from build123d import *

# Parameters (mm, degrees)
F0_W     = 18.8
F0_H     = 22.5
F1_DEPTH = 40


with BuildPart() as f1:
    # F0 (on Top) → F1 (new body)
    with BuildSketch(Plane.XY):
        Rectangle(F0_W, F0_H)
    extrude(amount=F1_DEPTH)

    # F2 (on Front) → F3 (revolve)
    with BuildSketch(Plane.XZ):
        Polygon((7.063377, 64.2), (0, 64.2), (0, 40), (9.4, 40), (9.4, 53.229246), (7.063377, 53.229246), align=None)
    revolve(axis=Axis((0, 0, 52.1), (0, 0, -1)))

    # F4 (on Front) → F5 (revolve)
    with BuildSketch(Plane.XZ):
        Polygon((11.3, 13.9), (9.4, 13.9), (9.4, 11.2), (19.2, 11.2), (19.2, 13), (11.3, 13), align=None)
        Polygon((-19.2, 11.2), (-9.4, 11.2), (-9.4, 13.9), (-11.3, 13.9), (-11.3, 13), (-19.2, 13), align=None)
    revolve(axis=Axis((-0.119775, 0, 11.2), (1, 0, 0)))


solid = f1.part
Work out the finished part from the listing and answer in its coordinate system (mm). A direction names the side the tool comes from. Give positions to 0.01 mm unless a question says otherwise; leave off trailing zeros. Write each loop counter-clockwise with the first axis right and the second up, starting at its lowest first coordinate (ties: lowest second). Pieces come first, ordered by that corner, then holes.
Q1. The part is cut by section D-D on y = -8.75. Give the vertices of the cut face in (x, z), and give its area (3 significant figures).
Answer:
outline: (-9.4, 0) - (9.4, 0) - (9.4, 40) - (3.43, 40) - (3.43, 53.23) - (-3.43, 53.23) - (-3.43, 40) - (-9.4, 40) - close
area: 843 mm2
Q2. The part is cut by section C-C on z = 11.2. Give the vertices of the cut face in (x, y), and give its area (3 significant figures).
Answer:
outline: (-19.2, -1.8) - (-11.3, -1.8) - (-11.3, -2.7) - (-9.4, -2.7) - (-9.4, -11.25) - (9.4, -11.25) - (9.4, -2.7) - (11.3, -2.7) - (11.3, -1.8) - (19.2, -1.8) - (19.2, 1.8) - (11.3, 1.8) - (11.3, 2.7) - (9.4, 2.7) - (9.4, 11.25) - (-9.4, 11.25) - (-9.4, 2.7) - (-11.3, 2.7) - (-11.3, 1.8) - (-19.2, 1.8) - close
area: 500 mm2
Q3. A tool of negligible diameter and unlimited length cuts with its end or side. For faces 1 (the face through (6.737, -2.122, 58.791)), 2 (the face through (10.337, 1.643, 9.057)), 3 (the face through (-1, -10, 40)), 4 (the face through (-10.363, 1.643, 9.057)), from which of +Z, -Z, +X, -X, +Y, -Y can it reach the whole face along a straight path? Write none if from no direction.
Answer:
face 1: +Z
face 2: +X
face 3: +Z, -Y
face 4: -X
Q4. The part is cut by section B-B on y = -4. Give the vertices of the cut face in (x, z), and give its area (3 significant figures).
Answer:
outline: (-9.4, 0) - (9.4, 0) - (9.4, 40) - (8.51, 40) - (8.51, 53.23) - (5.82, 53.23) - (5.82, 64.2) - (-5.82, 64.2) - (-5.82, 53.23) - (-8.51, 53.23) - (-8.51, 40) - (-9.4, 40) - close
area: 1,100 mm2
Q5. Straight lines are drawn through the part: L1, parallel to X at y = 1, z = 23; L2, parallel to Z at x = 1.5, y = 9.75; L3, parallel to Z at x = -8.5, y = 0. For each, find the intervals that lie inside material, in ascending order.
Answer:
L1: x = -9.4 to 9.4
L2: z = 0 to 40
L3: z = 0 to 53.23
Q6. Given pin 1 (10 mm diameter, centred on y = 8.5, z = 28, fed in from +X); pin 2 (1.5 mm diameter, centred on x = 6.5, y = 6, fed in from +Z); pin 3 (1.5 mm diameter, centred on y = 5, z = 13, fed in from -X), each flat-ended and moving along its own axis, determine where each tip first touches the part or whether it passes through.
Answer:
pin 1: stops at x = 9.4
pin 2: stops at z = 53.23
pin 3: stops at x = -9.4
Q7. The part is cut by section A-A on x = 0. Give the vertices of the cut face in (y, z).
Answer:
outline: (-11.25, 0) - (11.25, 0) - (11.25, 40) - (9.4, 40) - (9.4, 53.23) - (7.06, 53.23) - (7.06, 64.2) - (-7.06, 64.2) - (-7.06, 53.23) - (-9.4, 53.23) - (-9.4, 40) - (-11.25, 40) - close
